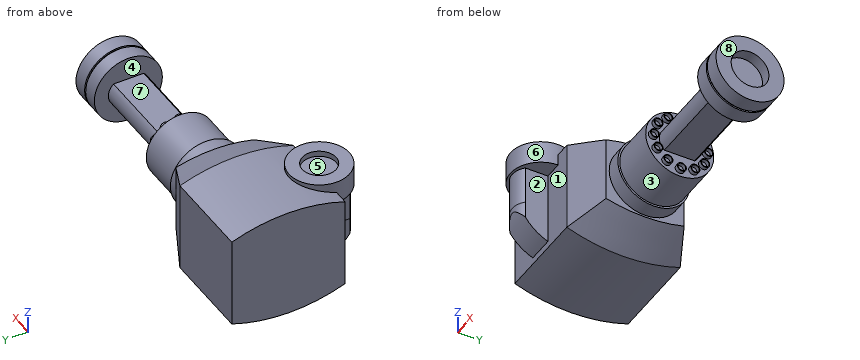
from build123d import *

# Parameters (mm, degrees)
BOSS_EXTRUDE1_DEPTH  = 30.48
BOSS_EXTRUDE2_DEPTH  = 12.7
BOSS_EXTRUDE2_DRAFT  = 25
SKETCH9_R            = 12.065
BOSS_EXTRUDE3_DEPTH  = 5.08
SKETCH10_R           = 11.43
BOSS_EXTRUDE4_DEPTH  = 15.24
SKETCH12_R           = 1.524
SKETCH12_R_2         = 1.27
BOSS_EXTRUDE6_DEPTH  = 1.27
CIRPATTERN2_COUNT    = 12
BOSS_EXTRUDE7_DEPTH  = 30.48
SKETCH14_R           = 11.43
BOSS_EXTRUDE8_DEPTH  = 5.08
SKETCH15_R           = 10.922
BOSS_EXTRUDE9_DEPTH  = 0.635
SKETCH16_R           = 11.43
BOSS_EXTRUDE10_DEPTH = 5.08
SKETCH17_R           = 10.16
BOSS_EXTRUDE14_DEPTH = 3.81
BOSS_EXTRUDE15_DEPTH = 12.7
BOSS_EXTRUDE16_DEPTH = 8.89
CUT_EXTRUDE1_DEPTH   = 8.89
SKETCH22_R           = 6.35
CUT_EXTRUDE2_DEPTH   = 3.81
SKETCH23_R           = 5.715
CUT_EXTRUDE4_DEPTH   = 1.905


with BuildPart() as part:
    # Sketch2 → Boss-Extrude1 (new body)
    with BuildSketch(Plane(origin=(0, 0, 0), x_dir=(0, 0, -1), z_dir=(1, 0, 0))):
        with BuildLine():
            Line((-15.24, 19.05), (15.24, 19.05))
            ThreePointArc((15.24, 19.05), (18.613103307, 0), (15.24, -19.05))
            Line((15.24, -19.05), (-15.24, -19.05))
            ThreePointArc((-15.24, -19.05), (-18.613103307, 0), (-15.24, 19.05))
        make_face()
    extrude(amount=BOSS_EXTRUDE1_DEPTH)


with BuildPart() as boss_extrude2_tool:
    # Sketch8 → Boss-Extrude2 (with draft: the straight prism first)
    with BuildSketch(Plane(origin=(30.48, 0, 0), x_dir=(0, 0, -1), z_dir=(1, 0, 0))):
        with BuildLine():
            Line((15.24, 19.05), (-15.24, 19.05))
            ThreePointArc((-15.24, 19.05), (-18.613103307, 0), (-15.24, -19.05))
            Line((-15.24, -19.05), (15.24, -19.05))
            ThreePointArc((15.24, -19.05), (18.613103307, 0), (15.24, 19.05))
        make_face()
    extrude(amount=BOSS_EXTRUDE2_DEPTH)
    # Boss-Extrude2: the draft: its side faces are tilted about the plane it starts from
    boss_extrude2_sides = [boss_extrude2_tool.faces().sort_by_distance(p)[0] for p in [
        (36.83, 19.05, 0),
        (36.83, 0, 18.613103307),
        (36.83, -19.05, 0),
        (36.83, 0, -18.613103307),
    ]]
    draft(boss_extrude2_sides, Plane(origin=(30.48, 0, 0), x_dir=(0, 0, -1), z_dir=(1, 0, 0)), BOSS_EXTRUDE2_DRAFT)


with BuildPart() as part_1:
    add(part.part)

    # Boss-Extrude2: add boss_extrude2_tool
    add(boss_extrude2_tool.part)

    # Sketch9 → Boss-Extrude3 (add)
    with BuildSketch(Plane(origin=(43.18, 0, 0), x_dir=(0, 0, -1), z_dir=(1, 0, 0))):
        Circle(SKETCH9_R)
    extrude(amount=BOSS_EXTRUDE3_DEPTH)

    # Sketch10 → Boss-Extrude4 (add)
    with BuildSketch(Plane(origin=(48.26, 0, 0), x_dir=(0, 0, -1), z_dir=(1, 0, 0))):
        Circle(SKETCH10_R)
    extrude(amount=BOSS_EXTRUDE4_DEPTH)

    # Sketch12 → Boss-Extrude6 (add)
    with BuildSketch(Plane(origin=(63.5, 0, 0), x_dir=(0, 0, -1), z_dir=(1, 0, 0))):
        with Locations((8.89, 0)):
            Circle(SKETCH12_R)
        with Locations((8.89, 0)):
            Circle(SKETCH12_R_2, mode=Mode.SUBTRACT)
    boss_extrude6 = extrude(amount=BOSS_EXTRUDE6_DEPTH)

    # CirPattern2: Boss-Extrude6 ×12 about axis
    cirpattern2_axis = Axis((0, 0, 0.160904977), (1, 0, 0))
    for i in range(1, CIRPATTERN2_COUNT):
        add(boss_extrude6.rotate(cirpattern2_axis, i * 360 / CIRPATTERN2_COUNT))

    # Sketch13 → Boss-Extrude7 (add)
    with BuildSketch(Plane(origin=(63.5, 0, 0), x_dir=(0, 0, -1), z_dir=(1, 0, 0))):
        with BuildLine():
            Line((3.81, 5.000460116), (3.81, -5.159539884))
            ThreePointArc((3.81, -5.159539884), (0, -6.879435719), (-3.81, -5.159539884))
            Line((-3.81, -5.159539884), (-3.81, 5.000460116))
            ThreePointArc((-3.81, 5.000460116), (0, 6.720355951), (3.81, 5.000460116))
        make_face()
    extrude(amount=BOSS_EXTRUDE7_DEPTH)

    # Sketch14 → Boss-Extrude8 (add)
    with BuildSketch(Plane(origin=(93.98, 0, 0), x_dir=(0, 0, -1), z_dir=(1, 0, 0))):
        Circle(SKETCH14_R)
    extrude(amount=BOSS_EXTRUDE8_DEPTH)

    # Sketch15 → Boss-Extrude9 (add)
    with BuildSketch(Plane(origin=(99.06, 0, 0), x_dir=(0, 0, -1), z_dir=(1, 0, 0))):
        Circle(SKETCH15_R)
    extrude(amount=BOSS_EXTRUDE9_DEPTH)

    # Sketch16 → Boss-Extrude10 (add)
    with BuildSketch(Plane(origin=(99.695, 0, 0), x_dir=(0, 0, -1), z_dir=(1, 0, 0))):
        Circle(SKETCH16_R)
    extrude(amount=BOSS_EXTRUDE10_DEPTH)

    # Sketch17 → Boss-Extrude14 (add, symmetric)
    with BuildSketch(Plane.XY.offset(15.24)):
        with Locations((15.24, -19.05)):
            Circle(SKETCH17_R)
    extrude(amount=BOSS_EXTRUDE14_DEPTH, both=True)

    # Sketch19 → Boss-Extrude15 (add)
    with BuildSketch(Plane(origin=(0, 0, 11.43), x_dir=(-1, 0, 0), z_dir=(0, 0, -1))):
        with BuildLine():
            Line((-19.418499269, -19.05), (-10.527211987, -19.05))
            Line((-10.527211987, -19.05), (-10.527211987, -26.67))
            ThreePointArc((-10.527211987, -26.67), (-14.972855628, -28.51144589), (-19.418499269, -26.67))
            Line((-19.418499269, -26.67), (-19.418499269, -19.05))
        make_face()
    extrude(amount=BOSS_EXTRUDE15_DEPTH)

    # Sketch20 → Boss-Extrude16 (add)
    with BuildSketch(Plane(origin=(19.418499269, 0, 0), x_dir=(0, 0, -1), z_dir=(1, 0, 0))):
        with BuildLine():
            Line((1.27, -19.05), (12.926323027, -19.05))
            ThreePointArc((12.926323027, -19.05), (8.330590053, -25.484349932), (1.27, -29.043800552))
            Line((1.27, -29.043800552), (1.27, -19.05))
        make_face()
    extrude(amount=-BOSS_EXTRUDE16_DEPTH)

    # Sketch21 → Cut-Extrude1 (cut)
    with BuildSketch(Plane.XY.offset(-1.27)):
        with BuildLine():
            Line((10.528499269, -26.671286909), (10.528499269, -29.043800552))
            Line((10.528499269, -29.043800552), (19.418499269, -29.043800552))
            Line((19.418499269, -29.043800552), (19.418499269, -26.67))
            ThreePointArc((19.418499269, -26.67), (14.973765742, -28.511445824), (10.528499269, -26.671286909))
        make_face()
    extrude(amount=-CUT_EXTRUDE1_DEPTH, mode=Mode.SUBTRACT)

    # Sketch22 → Cut-Extrude2 (cut)
    with BuildSketch(Plane(origin=(104.775, 0, 0), x_dir=(0, 0, -1), z_dir=(1, 0, 0))):
        Circle(SKETCH22_R)
    extrude(amount=-CUT_EXTRUDE2_DEPTH, mode=Mode.SUBTRACT)

    # Sketch23 → Cut-Extrude4 (cut)
    with BuildSketch(Plane.XY.offset(19.05)):
        with Locations((15.24, -19.05)):
            Circle(SKETCH23_R)
    extrude(amount=-CUT_EXTRUDE4_DEPTH, mode=Mode.SUBTRACT)


solid = part_1.part
The listing builds one solid part. Answer for the finished solid, in the listing's coordinates (mm). Face numbers are marked on the shaded views. A direction names the side the tool comes from. Round coordinates to 2 decimals unless told otherwise and drop trailing zeros. Write each loop counter-clockwise with the first axis right and the second up, starting at its lowest first coordinate (ties: lowest second). Pieces come first, ordered by that corner, then holes. Notation, with made-up numbers: (40.25, 67.5) - (72.25, 67.5) arc R16 ccw to (72.25, 82.5) - close; hole circle Ø6 at (43.5, -33.75). An arc over 180 degrees is marked (long way). Use a Markdown table: item, result. Add a question column.
1. Flat-ended cylindrical pins translate along their axes: P1, Ø3.5, axis at y = 0, z = -8.89, coming from the -X side; P2, Ø4, axis at x = 23.5, y = -7.5, coming from the +Z side; P3, Ø2, axis at x = 91, z = 7, coming from the +Y side; P4, Ø4, axis at y = -23, z = 6, coming from the -X side. Find the tip coordinate at first contact, or state that the pin passes through.
2. The part is cut by section C-C (x = 91.5). Write down the section's boundary in (y, z).
3. A tool of negligible diameter and unlimited length cuts with its end or side. For the marked faces 1, 2, 3, 4 and 5, from which of +Z, -Z, +X, -X, +Y, -Y can it reach the whole face along a straight path? Write none if from no direction.
4. The part is cut by section A-A (x = 12.5). Write down the section's boundary in (y, z) (3 decimals).
5. Consider line 1 (Y direction, x = 22.5, z = -5); line 2 (X direction, y = -13, z = 1.5). Determine where each line is inside the solid, lowest interval first.
6. For a pull along X with two mould halves and no side action, classify the marked faces 6, 7 and 8 as +X half, -X half, draft (parallel to the pull), parting line (faces both ways), or undercut.
7. The part is cut by section B-B (x = 24). Write down the section's boundary in (y, z), and give its area (3 significant figures).
Reported:
| question | item | result |
|---|---|---|
| 1 | P1 | x = 0 |
| 1 | P2 | z = 18.34 |
| 1 | P3 | through |
| 1 | P4 | x = 10.53 |
| 2 | outline | (-5.16, -3.81) - (5, -3.81) arc R5.08 ccw to (5, 3.81) - (-5.16, 3.81) arc R5.08 ccw to start |
| 3 | face 1 | -Z, -Y |
| 3 | face 2 | -Z, +X, -Y |
| 3 | face 3 | +X |
| 3 | face 4 | none |
| 3 | face 5 | +Z |
| 4 | outline | (-28.834, 11.43) - (-28.005, 11.43) - (-28.005, -4.363) arc R16.51 ccw to (-19.05, -12.926) - (-19.05, -15.24) arc R55.48 ccw to (19.05, -15.24) - (19.05, 15.24) arc R55.48 ccw to (-9.266, 17.834) - (-9.266, 19.05) - (-14.035, 19.05) - (-14.035, 17.145) - (-24.065, 17.145) - (-24.065, 19.05) - (-28.834, 19.05) - close |
| 5 | line 1 | -19.05 to 19.05 |
| 5 | line 2 | 0 to 43.18 |
| 6 | face 6 | parting line |
| 6 | face 7 | undercut |
| 6 | face 8 | +X half |
| 7 | outline | (-24.2, 11.43) - (-19.05, 11.43) - (-19.05, -15.24) arc R55.48 ccw to (19.05, -15.24) - (19.05, 15.24) arc R55.48 ccw to (-13.9, 16.84) - (-13.9, 19.05) - (-24.2, 19.05) - close |
| 7 | area | 1,390 mm^2 |
